Study the drawing (mm; zero at the part's minimum x, y, z) and answer. A direction names the side the tool comes from. Round coordinates to 2 decimals unless told otherwise and drop trailing zeros. Order: outer loops, then holes, each group sorted by start corner. A loop starts at its lowest first (then second) coordinate and runs counter-clockwise, first axis right, second up. Notation, with made-up numbers: M 14,37.5 L 26,37.5 A25 cw 26,66.5 Z; hole C 74,39 d8. An arc over 180 degrees is marked long. Put each result on its own line as item: value. Start each with the question number.
1. Which of the six approach directions +Z, -Z, +X, -X, +Y, -Y give full straight-line access (tool end or side, diameter ignored) to the marked faces 1 and 2?
2. Each of these flat-tipped pins is pushed along its axis until it touches: pin 1 Ø5 at (x, y) = (7, 8) entering from -Z; pin 2 Ø2 at (x, y) = (14, 4) entering from +Z; pin 3 Ø1 at (x, z) = (8, 5) entering from +Y; pin 4 Ø3.5 at (y, z) = (6.5, 7) entering from -X. Where does it stop, or does it pass through?
3. The part is cut by section C-C (x = 22.5). Give the vertices of the cut face in (y, z) (3 decimals), then the cut area to 3 significant figures.
4. Consider line 1 (Y direction, x = 8.75, z = 5.6); line 2 (Y direction, x = 13, z = 5.6) (3 decimals); line 3 (Z direction, x = 21.75, y = 5.75). Determine where each line is inside the solid, lowest interval first.
5. The mould has two halves that part along Y. Classify the marked faces 3 and 4: +Y half, -Y half, draft (parallel to the pull), parting line (faces both ways), or undercut.
6. The part is cut by section A-A (z = 5.6). Give the vertices of the cut face in (x, y) (3 decimals).
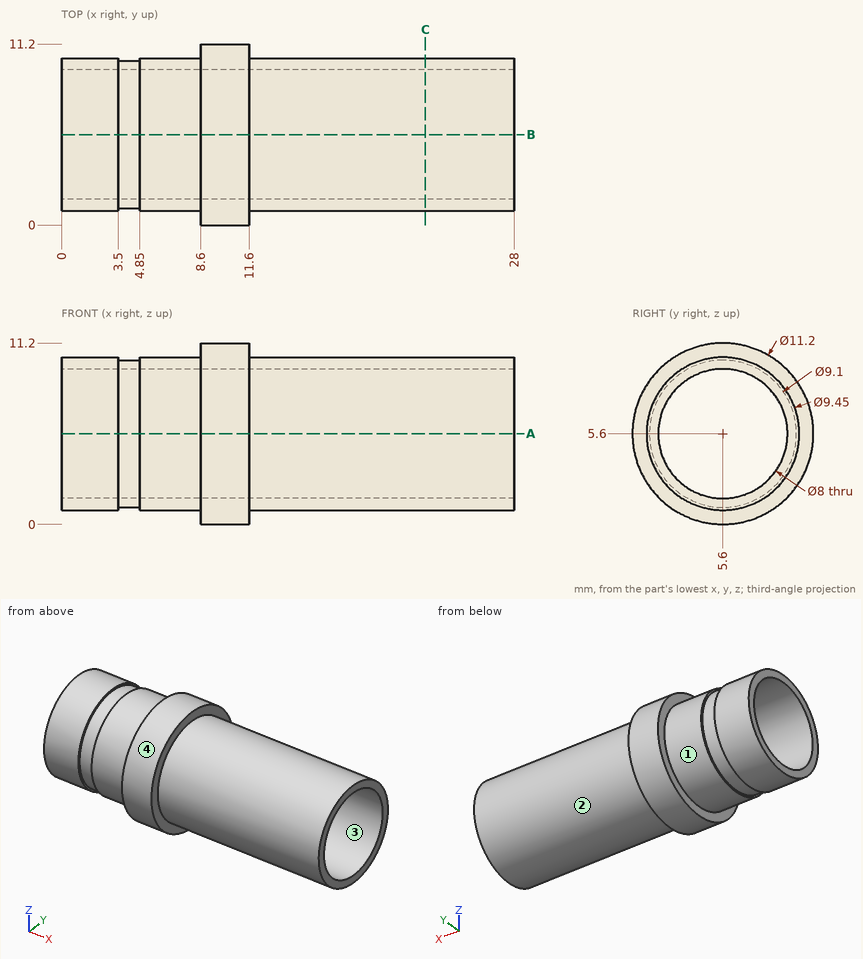
Resolved:
1. face 1: -X
1. face 2: +X
2. pin 1: z = 0.02
2. pin 2: z = 10.29
2. pin 3: y = 10.32
2. pin 4: through
3. outline: C 5.6,5.6 d9.45; hole C 5.6,5.6 d8
3. area: 19.9 mm2
4. line 1: 0 to 1.6, 9.6 to 11.2
4. line 2: 0.875 to 1.6, 9.6 to 10.325
4. line 3: 0.88 to 1.6, 9.6 to 10.32
5. face 3: undercut
5. face 4: parting line
6. outline: M 0,0.875 L 3.5,0.875 L 3.5,1.05 L 4.85,1.05 L 4.85,0.875 L 8.6,0.875 L 8.6,0 L 11.6,0 L 11.6,0.875 L 28,0.875 L 28,1.6 L 0,1.6 Z; M 0,9.6 L 28,9.6 L 28,10.325 L 11.6,10.325 L 11.6,11.2 L 8.6,11.2 L 8.6,10.325 L 4.85,10.325 L 4.85,10.15 L 3.5,10.15 L 3.5,10.325 L 0,10.325 Z
